```python
from build123d import *

# Parameters (mm, degrees)
F0_W     = 152.4
F0_H     = 76.2
F0_R     = 6.35
F1_DEPTH = 12.7
F2_R     = 5.08
F3_W     = 38.1
F3_H     = 76.2
F4_DEPTH = 12.7


with BuildPart() as f1:
    # F0 (on Front) → F1 (new body)
    with BuildSketch(Plane.XZ):
        with Locations((-0.517488, -6.741711)):
            Rectangle(F0_W, F0_H)
        with Locations((-64.017488, -25.791711)):
            Circle(F0_R, mode=Mode.SUBTRACT)
        with Locations((62.982512, -25.791711)):
            Circle(F0_R, mode=Mode.SUBTRACT)
        with Locations((-64.017488, 12.308289)):
            Circle(F0_R, mode=Mode.SUBTRACT)
        with Locations((62.982512, 12.308289)):
            Circle(F0_R, mode=Mode.SUBTRACT)
    extrude(amount=F1_DEPTH)

    # F2
    f2_edges = [f1.edges().sort_by_distance(p)[0] for p in [
        (-76.717488, -6.35, 31.358289),
        (-76.717488, -6.35, -44.841711),
        (75.682512, -6.35, -44.841711),
        (75.682512, -6.35, 31.358289),
    ]]
    fillet(f2_edges, radius=F2_R)

    # F3 (on face) → F4 (join)
    with BuildSketch(Plane.XZ.offset(12.7)):
        with Locations((-57.667488, -6.741711)):
            Rectangle(F3_W, F3_H)
    extrude(amount=F4_DEPTH)


solid = f1.part
```
Design review of the part built by this model. Coordinates are the model's own, in mm. A direction names the side the tool comes from. Give positions to 0.01 mm unless a question says otherwise; leave off trailing zeros. Order: outer loops, then holes, each group sorted by start corner. A loop starts at its lowest first (then second) coordinate and runs counter-clockwise, first axis right, second up. Notation, with made-up numbers: (89, -16.75) - (105, -16.75) arc R7 cw to (105, -11.75) - close; hole circle Ø7 at (-3.75, 54). An arc over 180 degrees is marked (long way). Use a Markdown table: item, result. Add a question column.
(1) Wall thickness on probe 1 along X at (y, z) = (-8.5, -30); probe 2 along Y at (x, z) = (69.5, -38); probe 3 along X at (y, z) = (-24, 23): over which ranges is each line inside the solid? List them lowest first. Write a range as [from, to].
(2) Add section B-B on y = -11.25. Give the boundary of the cut face in (x, z).
(3) Clearance check with flat-ended pins moving along their axes: P1, Ø4, axis at x = -7, z = 6.5, coming from the -Y side; P2, Ø4, axis at x = -63, z = -23, coming from the +Y side. State where each tip first meets the part, or that it passes through.
(4) Mouldability with a two-part tool opening along Z and no side actions: class faces 5 (the face through (75.683, -6, -7)), 6 (the face through (-75.3, -6.4, 29.8)), 7 (the face through (-64, -12.7, -26)) as +Z half, -Z half, draft (parallel to the pull), parting line (faces both ways), or undercut.
(5) Add section D-D on z = -30.5. Give the boundary of the cut face in (x, y).
(6) Add section A-A on z = -22.5. Give the boundary of the cut face in (x, y), then the cut area to 3 significant figures.
(7) Add section C-C on x = -21. Give the boundary of the cut face in (y, z), then the cut area to 3 significant figures.
(8) Machinability: for faces 1 (the face through (-76, -12.7, -44)), 2 (the face through (-76, -12.7, 30)), 3 (the face through (-58.15, -6.26, 9.88)), 4 (the face through (-38.617, -19, -7)), which of the approach directions +Z, -Z, +X, -X, +Y, -Y give a long, thin tool a straight path to every point of the face, cutting with its end or side? Answer none if there is none.
Report:
| question | item | result |
|---|---|---|
| 1 | probe 1 | x = [-76.72, -68.77], [-59.26, 58.23], [67.74, 75.68] |
| 1 | probe 2 | y = [-12.7, 0] |
| 1 | probe 3 | x = [-76.72, -38.62] |
| 2 | outline | (-76.72, -39.76) arc R5.08 ccw to (-71.64, -44.84) - (70.6, -44.84) arc R5.08 ccw to (75.68, -39.76) - (75.68, 26.28) arc R5.08 ccw to (70.6, 31.36) - (-71.64, 31.36) arc R5.08 ccw to (-76.72, 26.28) - close; hole circle Ø12.7 at (-64.02, -25.79); hole circle Ø12.7 at (-64.02, 12.31); hole circle Ø12.7 at (62.98, -25.79); hole circle Ø12.7 at (62.98, 12.31) |
| 3 | P1 | stops at y = -12.7 |
| 3 | P2 | stops at y = -12.7 |
| 4 | face 5 | draft |
| 4 | face 6 | +Z half |
| 4 | face 7 | undercut |
| 5 | outline | (-76.72, -25.4) - (-38.62, -25.4) - (-38.62, -12.7) - (58.72, -12.7) - (58.72, 0) - (-59.76, 0) - (-59.76, -12.7) - (-68.28, -12.7) - (-68.28, 0) - (-76.72, 0) - close; (67.24, -12.7) - (75.68, -12.7) - (75.68, 0) - (67.24, 0) - close |
| 6 | outline | (-76.72, -25.4) - (-38.62, -25.4) - (-38.62, -12.7) - (57.55, -12.7) - (57.55, 0) - (-58.59, 0) - (-58.59, -12.7) - (-69.45, -12.7) - (-69.45, 0) - (-76.72, 0) - close; (68.41, -12.7) - (75.68, -12.7) - (75.68, 0) - (68.41, 0) - close |
| 6 | area | 2,140 mm² |
| 7 | outline | (-12.7, -44.84) - (0, -44.84) - (0, 31.36) - (-12.7, 31.36) - close |
| 7 | area | 968 mm² |
| 8 | face 1 | -Z, -X, +Y |
| 8 | face 2 | +Z, -X, +Y |
| 8 | face 3 | +Y |
| 8 | face 4 | +Z, -Z, +X, -Y |
